from build123d import *

# Parameters (mm, degrees)
SKETCH1_W                      = 75
SKETCH1_H                      = 200
BASE_FLANGE1_DEPTH             = 2
EDGE_FLANGE1_STRIP_W           = 10
EDGE_FLANGE1_STRIP_H           = 2
EDGE_FLANGE1_STRIP_CUT_DEPTH   = 75
EDGE_FLANGE1_STRIP_2_W         = 10
EDGE_FLANGE1_STRIP_2_H         = 2
EDGE_FLANGE1_STRIP_CUT_2_DEPTH = 75
EDGE_FLANGE1_DEPTH             = 75
EDGE_FLANGE1_BEND_DEPTH        = 75
EDGE_FLANGE2_STRIP_W           = 10
EDGE_FLANGE2_STRIP_H           = 2
EDGE_FLANGE2_STRIP_CUT_DEPTH   = 75
EDGE_FLANGE2_STRIP_2_W         = 10
EDGE_FLANGE2_STRIP_2_H         = 2
EDGE_FLANGE2_STRIP_CUT_2_DEPTH = 75
EDGE_FLANGE2_DEPTH             = 75
EDGE_FLANGE2_BEND_DEPTH        = 75
SKETCH18_R                     = 4.6
CUT_EXTRUDE1_DEPTH             = 10
SKETCH19_R                     = 4.6
CUT_EXTRUDE2_DEPTH             = 10
SKETCH20_R                     = 4.6
CUT_EXTRUDE3_DEPTH             = 10


# Sheet-metal steps are written as plain solids
with BuildPart() as part:
    # Sketch1 → Base-Flange1 (new body)
    with BuildSketch(Plane(origin=(0, 0, 0), x_dir=(0, 0, -1), z_dir=(1, 0, 0))):
        Rectangle(SKETCH1_W, SKETCH1_H)
    extrude(amount=-BASE_FLANGE1_DEPTH)

    # Edge-Flange1 strip (across the edge) → Edge-Flange1 strip cut (cut)
    with BuildSketch(Plane(origin=(0, 100, -37.5), x_dir=(0, -1, 0), z_dir=(0, 0, 1))):
        with Locations((-2, -1)):
            Rectangle(EDGE_FLANGE1_STRIP_W, EDGE_FLANGE1_STRIP_H)
    extrude(amount=EDGE_FLANGE1_STRIP_CUT_DEPTH, mode=Mode.SUBTRACT)

    # Edge-Flange1 strip 2 (across the edge) → Edge-Flange1 strip cut 2 (cut)
    with BuildSketch(Plane(origin=(-2, -100, -37.5), x_dir=(0, 1, 0), z_dir=(0, 0, 1))):
        with Locations((-2, -1)):
            Rectangle(EDGE_FLANGE1_STRIP_2_W, EDGE_FLANGE1_STRIP_2_H)
    extrude(amount=EDGE_FLANGE1_STRIP_CUT_2_DEPTH, mode=Mode.SUBTRACT)

    # Edge-Flange1 section (across the edge) → Edge-Flange1 (add)
    with BuildSketch(Plane(origin=(0, 100, -37.5), x_dir=(0, -1, 0), z_dir=(0, 0, 1))):
        with BuildLine():
            Line((0, 1), (0, 46))
            Line((0, 46), (2, 46))
            Line((2, 46), (2, 1))
            ThreePointArc((2, 1), (2.292893219, 0.292893219), (3, 0))
            Line((3, 0), (3, -2))
            ThreePointArc((3, -2), (0.878679656, -1.121320344), (0, 1))
        make_face()
    extrude(amount=EDGE_FLANGE1_DEPTH)

    # Edge-Flange1 section 2 (across the edge) → Edge-Flange1 bend (add)
    with BuildSketch(Plane(origin=(-2, -100, -37.5), x_dir=(0, 1, 0), z_dir=(0, 0, 1))):
        with BuildLine():
            Line((0, 1), (0, 46))
            Line((0, 46), (2, 46))
            Line((2, 46), (2, 1))
            ThreePointArc((2, 1), (2.292893219, 0.292893219), (3, 0))
            Line((3, 0), (3, -2))
            ThreePointArc((3, -2), (0.878679656, -1.121320344), (0, 1))
        make_face()
    extrude(amount=EDGE_FLANGE1_BEND_DEPTH)

    # Edge-Flange2 strip (across the edge) → Edge-Flange2 strip cut (cut)
    with BuildSketch(Plane(origin=(46, 98, -37.5), x_dir=(-1, 0, 0), z_dir=(0, 0, 1))):
        with Locations((-2, -1)):
            Rectangle(EDGE_FLANGE2_STRIP_W, EDGE_FLANGE2_STRIP_H)
    extrude(amount=EDGE_FLANGE2_STRIP_CUT_DEPTH, mode=Mode.SUBTRACT)

    # Edge-Flange2 strip 2 (across the edge) → Edge-Flange2 strip cut 2 (cut)
    with BuildSketch(Plane(origin=(-48, -98, -37.5), x_dir=(1, 0, 0), z_dir=(0, 0, 1))):
        with Locations((-2, -1)):
            Rectangle(EDGE_FLANGE2_STRIP_2_W, EDGE_FLANGE2_STRIP_2_H)
    extrude(amount=EDGE_FLANGE2_STRIP_CUT_2_DEPTH, mode=Mode.SUBTRACT)

    # Edge-Flange2 section (across the edge) → Edge-Flange2 (add)
    with BuildSketch(Plane(origin=(46, 98, -37.5), x_dir=(-1, 0, 0), z_dir=(0, 0, 1))):
        with BuildLine():
            Line((0, 1), (0, 21))
            Line((0, 21), (2, 21))
            Line((2, 21), (2, 1))
            ThreePointArc((2, 1), (2.292893219, 0.292893219), (3, 0))
            Line((3, 0), (3, -2))
            ThreePointArc((3, -2), (0.878679656, -1.121320344), (0, 1))
        make_face()
    extrude(amount=EDGE_FLANGE2_DEPTH)

    # Edge-Flange2 section 2 (across the edge) → Edge-Flange2 bend (add)
    with BuildSketch(Plane(origin=(-48, -98, -37.5), x_dir=(1, 0, 0), z_dir=(0, 0, 1))):
        with BuildLine():
            Line((0, 1), (0, 21))
            Line((0, 21), (2, 21))
            Line((2, 21), (2, 1))
            ThreePointArc((2, 1), (2.292893219, 0.292893219), (3, 0))
            Line((3, 0), (3, -2))
            ThreePointArc((3, -2), (0.878679656, -1.121320344), (0, 1))
        make_face()
    extrude(amount=EDGE_FLANGE2_BEND_DEPTH)

    # Sketch18 → Cut-Extrude1 (cut)
    with BuildSketch(Plane(origin=(0, 100, 0), x_dir=(1, 0, 0), z_dir=(0, 1, 0))):
        with Locations(Location((21, 0, 0), (0, 0, 180))):
            Circle(SKETCH18_R)
    extrude(amount=-CUT_EXTRUDE1_DEPTH, mode=Mode.SUBTRACT)

    # Sketch19 → Cut-Extrude2 (cut)
    with BuildSketch(Plane(origin=(0, -98, 0), x_dir=(1, 0, 0), z_dir=(0, 1, 0))):
        with Locations(Location((-23, 0, 0), (0, 0, 180))):
            Circle(SKETCH19_R)
    extrude(amount=-CUT_EXTRUDE2_DEPTH, mode=Mode.SUBTRACT)

    # Sketch20 → Cut-Extrude3 (cut)
    with BuildSketch(Plane(origin=(0, 0, 0), x_dir=(0, 0, -1), z_dir=(1, 0, 0))):
        with Locations((0, -64)):
            Circle(SKETCH20_R)
    extrude(amount=-CUT_EXTRUDE3_DEPTH, mode=Mode.SUBTRACT)


solid = part.part
Model file for the job. Use its own axes, mm. A direction names the side the tool comes from. Give positions to 0.01 mm unless a question says otherwise; leave off trailing zeros. Order: outer loops, then holes, each group sorted by start corner. A loop starts at its lowest first (then second) coordinate and runs counter-clockwise, first axis right, second up. Notation, with made-up numbers: (37.5, 13.25) - (74.5, 13.25) arc R20 cw to (74.5, 21.25) - close; hole circle Ø9 at (2, -29). An arc over 180 degrees is marked (long way). Return JSON: item names as keys, results as strings.
1) Cut at A-A, the plane y = 86.5. Give the cut face in (x, z).
Geometry says:
{"outline": "(-2, -37.5) - (0, -37.5) - (0, 37.5) - (-2, 37.5) - close; (44, -37.5) - (46, -37.5) - (46, 37.5) - (44, 37.5) - close"}
2) Cut at D-D, the plane x = -8. Give the cut face in (y, z), plus the area to 3 significant figures.
Geometry says:
{"outline": "(-100, -37.5) - (-98, -37.5) - (-98, 37.5) - (-100, 37.5) - close", "area": "150 mm²"}
3) Flat gauge pins, fed straight in: P1, Ø3, axis at x = -3, z = 16, coming from the +Y side; P2, Ø4, axis at y = -26, z = 29, coming from the +X side; P3, Ø1, axis at y = 11, z = -21.5, coming from the -X side. Where does each tip first touch, or does it go through?
Geometry says:
{"P1": "y = 98.66", "P2": "x = 0", "P3": "x = -2"}
4) Cut at C-C, the plane x = 21. Give the cut face in (y, z).
Geometry says:
{"outline": "(98, -37.5) - (100, -37.5) - (100, -4.6) - (98, -4.6) - close; (98, 4.6) - (100, 4.6) - (100, 37.5) - (98, 37.5) - close"}
5) Probe line 1 (Z direction, x = 21, y = 99.35); line 2 (X direction, y = -91.5, z = 13.5); line 3 (Y direction, x = -33.5, z = 3). List the from-to ranges inside material, lowest first. Write a range as from..to.
Geometry says:
{"line 1": "-37.5..-4.6, 4.6..37.5", "line 2": "-48..-46, -2..0", "line 3": "-100..-98"}
6) Pull direction X, two halves, no side cores. Call faces 4 (the flat face through (27, 98, -1)), 5 (the flat face through (-48, -87, -1)), 6 (the flat face through (-1, 0, -37.5)): pulls with the +X half, pulls with the -X half, needs draft (parallel to the pull), parting line crosses it, or undercut.
Geometry says:
{"face 4": "undercut", "face 5": "pulls with the -X half", "face 6": "needs draft"}
7) 3-axis set-ups, long thin cutter, end or side, ignore diameter. For faces 1 (the flat face through (44, 87, -1)), 2 (the flat face through (-46, -87, -1)), 3 (the flat face through (46, 87, -1)): which of +Z, -Z, +X, -X, +Y, -Y reach the whole face in a straight line?
Geometry says:
{"face 1": "+Z, -Z, -Y", "face 2": "+Z, -Z, +Y", "face 3": "+Z, -Z, +X, +Y, -Y"}
8) Cut at B-B, the plane z = 0. Count the separate pieces of the cut face and the enclosed holes in it, plus the area to 3 significant figures.
Geometry says:
{"separate pieces": "4", "enclosed holes": "0", "area": "606 mm²"}
